Check sheet for the modelled part. Datum: model origin and axes. Units: mm. Face numbers are marked on the shaded views. A direction names the side the tool comes from. Give positions to 0.01 mm unless a question says otherwise; leave off trailing zeros. Loops run counter-clockwise (first coordinate to the right, second up) from the corner with the lowest first, then second, coordinate; pieces in that order, holes last. Notation, with made-up numbers: (65, 82.25) - (81, 82.25) arc R30 cw to (81, 107.25) - close; hole circle Ø6 at (-36, 45). An arc over 180 degrees is marked (long way). Use one line per item in the form item = value.
from build123d import *

# Parameters (mm, degrees)
CUT_EXTRUDE1_DEPTH = 0.5


with BuildPart() as part:
    # Sketch1 → Revolve1 (revolve)
    with BuildSketch(Plane.XY):
        with BuildLine():
            Line((0, 0), (0, 2))
            Line((0, 2), (0.6, 2))
            Line((0.6, 2), (1.413030615, 1.084040821))
            ThreePointArc((1.413030615, 1.084040821), (1.497505597, 1.021976103), (1.6, 1))
            Line((1.6, 1), (6.579697282, 1))
            ThreePointArc((6.579697282, 1), (6.908495257, 0.972787848), (7.228345931, 0.891891892))
            Line((7.228345931, 0.891891892), (9.27789548, 0.189189189))
            ThreePointArc((9.27789548, 0.189189189), (9.37577731, 0.116247639), (9.413030615, 0))
            Line((9.413030615, 0), (0, 0))
        make_face()
    revolve(axis=Axis((-3.974685283, 0, 0), (1, 0, 0)))

    # Sketch2 → Cut-Extrude1 (cut)
    with BuildSketch(Plane.ZY):
        Polygon((-0.25, 1), (0.25, 1), (0.362422173, 0.362422173), (1, 0.25), (1, -0.25), (0.362422173, -0.362422173), (0.25, -1), (-0.25, -1), (-0.362422173, -0.362422173), (-1, -0.25), (-1, 0.25), (-0.362422173, 0.362422173), align=None)
    extrude(amount=-CUT_EXTRUDE1_DEPTH, mode=Mode.SUBTRACT)


solid = part.part
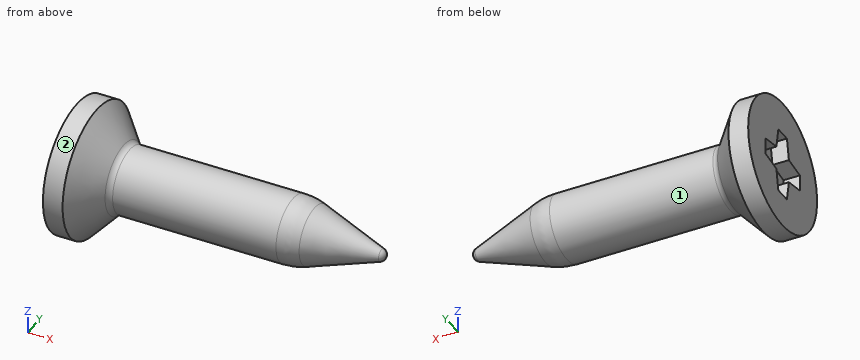
Item 1: Gauge pin test, flat ends, axial feed: P1, Ø1, axis at x = 2, y = 0, coming from the +Z side; P2, Ø2, axis at x = 2.5, z = 0, coming from the +Y side; P3, Ø2, axis at y = 0.5, z = -0.5, coming from the -X side. Record the tip position at first contact, or that the pin passes through.
Answer block:
P1 = 1.02
P2 = 1.02
P3 = 0
Item 2: Section check A-A on x = 2. Record the boundary of the cut face in (y, z), then the cut area to 3 significant figures.
Answer block:
outline = circle Ø2 at (0, 0)
area = 3.14 mm2
Item 3: Section check B-B on x = 8.5. Record the boundary of the cut face in (y, z), then the cut area to 3 significant figures.
Answer block:
outline = circle Ø0.91 at (0, 0)
area = 0.653 mm2
Item 4: Thickness scan on L1, parallel to Z at x = 4.25, y = 0.35; L2, parallel to Z at x = 6.25, y = -0.75; L3, parallel to Y at x = 1, z = -0.85. Record the ranges inside material, lowest first.
Answer block:
L1 = -0.94 to 0.94
L2 = -0.66 to 0.66
L3 = -1.3 to 1.3
Item 5: Access from +Z, -Z, +X, -X, +Y, -Y to the whole of each face (thin tool, end or side, straight path). Record for the marked faces 1 and 2.
Answer block:
face_1 = +X
face_2 = +X, -X
